For this review, take the finished solid that the model builds, in its own axes (mm). A direction names the side the tool comes from. Give positions to 0.01 mm unless a question says otherwise; leave off trailing zeros. Order: outer loops, then holes, each group sorted by start corner. A loop starts at its lowest first (then second) coordinate and runs counter-clockwise, first axis right, second up. Notation, with made-up numbers: M 55,-29.5 L 60,-29.5 A31 ccw 60,-3.5 Z; hole C -26,20.5 d2. An arc over 180 degrees is marked long. Use CSV: the item, a comma, the result in double quotes. Start each with the question number.
(1) Clearance check with flat-ended pins moving along their axes: P1, Ø4, axis at x = -5, z = 11, coming from the -Y side; P2, Ø6.5, axis at x = 15, z = -15, coming from the +Y side; P3, Ø2.5, axis at y = 3.5, z = -18, coming from the +X side. State where each tip first meets the part, or that it passes through.
(2) Draft analysis for pull direction Z (two halves, no side actions). For faces 4 (the face through (-23, 2, -25)), 5 (the face through (24.53, 2.54, 11.31)), 6 (the face through (-15.1, 2.5, -12.5)), 7 (the face through (-21, 2, 25)), state which applies: pulls with the +Z half, pulls with the -Z half, needs draft (parallel to the pull), parting line crosses it, or undercut.
(3) Tool access review of faces 1 (the face through (11.25, 2.535, -24.554)), 2 (the face through (18.69, 2.46, 24.53)), 3 (the face through (-25, 2, 2)): name each direction out of +Z, -Z, +X, -X, +Y, -Y from which nothing blocks a thin tool from reaching the whole face with its end or side.
(4) Consider section C-C (y = 3.65). Give the number of separate pieces and of enclosed holes in the cut face, and give its area (3 significant figures).
(5) Wall thickness on L1, parallel to X at y = 3.75, z = -15; L2, parallel to X at y = 1.4, z = 0; L3, parallel to Z at x = 0, y = 1.5: over which ranges is each line inside the solid? List them lowest first. Write a range as from..to.
(6) Consider section A-A (z = 16). Write out the cut boundary in (x, y).
(7) Consider section B-B (z = 3.5). Write out the cut boundary in (x, y).
```python
from build123d import *

# Parameters (mm, degrees)
SKETCH1_W           = 50
SKETCH1_H           = 50
SKETCH1_R           = 2.5
BOSS_EXTRUDE1_DEPTH = 5
SKETCH2_R           = 2.5
CUT_EXTRUDE1_DEPTH  = 5
CUT_EXTRUDE2_DEPTH  = 36.707142143
FILLET1_R           = 6


with BuildPart() as part:
    # Sketch1 → Boss-Extrude1 (new body)
    with BuildSketch(Plane(origin=(0, 0, 0), x_dir=(1, 0, 0), z_dir=(0, 1, 0))):
        Rectangle(SKETCH1_W, SKETCH1_H)
        with Locations(Location((15, 15, 0), (0, 0, 270))):
            Circle(SKETCH1_R, mode=Mode.SUBTRACT)
        with Locations(Location((15, -15, 0), (0, 0, 270))):
            Circle(SKETCH1_R, mode=Mode.SUBTRACT)
        with Locations(Location((-15, -15, 0), (0, 0, 90))):
            Circle(SKETCH1_R, mode=Mode.SUBTRACT)
        with Locations(Location((-15, 15, 0), (0, 0, 90))):
            Circle(SKETCH1_R, mode=Mode.SUBTRACT)
    extrude(amount=BOSS_EXTRUDE1_DEPTH)

    # Sketch2 → Cut-Extrude1 (cut)
    with BuildSketch(Plane(origin=(0, 5, 0), x_dir=(1, 0, 0), z_dir=(0, 1, 0))):
        with Locations((25, 15)):
            Circle(SKETCH2_R)
        with Locations((25, -15)):
            Circle(SKETCH2_R)
        with Locations((-25, 15)):
            Circle(SKETCH2_R)
        with Locations((-25, -15)):
            Circle(SKETCH2_R)
        with Locations((-15, 25)):
            Circle(SKETCH2_R)
        with Locations((15, 25)):
            Circle(SKETCH2_R)
        with Locations((15, -25)):
            Circle(SKETCH2_R)
        with Locations((-15, -25)):
            Circle(SKETCH2_R)
    extrude(amount=-CUT_EXTRUDE1_DEPTH, mode=Mode.SUBTRACT)

    # Sketch3 → Cut-Extrude2 (cut, through all)
    with BuildSketch(Plane(origin=(0, 5, 0), x_dir=(1, 0, 0), z_dir=(0, 1, 0))):
        with BuildLine():
            Line((-3, 19.696938457), (3, 19.696938457))
            Line((3, 19.696938457), (3, 14.696938457))
            ThreePointArc((3, 14.696938457), (0, -15), (-3, 14.696938457))
            Line((-3, 14.696938457), (-3, 19.696938457))
        make_face()
    extrude(amount=-CUT_EXTRUDE2_DEPTH, mode=Mode.SUBTRACT)

    # Fillet1
    fillet1_edges = [part.edges().sort_by_distance(p)[0] for p in [
        (-12.5, 2.5, 25),
        (17.5, 2.5, 25),
        (-25, 2.5, -12.5),
        (-25, 2.5, 17.5),
        (12.5, 2.5, -25),
        (-17.5, 2.5, -25),
        (25, 2.5, -17.5),
        (25, 2.5, 12.5),
    ]]
    fillet(fillet1_edges, radius=FILLET1_R)


solid = part.part
```
Check result:
1,P1,"passes through"
1,P2,"stops at y = 5"
1,P3,"stops at x = 24.73"
2,face 4,"pulls with the -Z half"
2,face 5,"undercut"
2,face 6,"undercut"
2,face 7,"pulls with the +Z half"
3,face 1,"-Z, +Y, -Y"
3,face 2,"+Z, +Y, -Y"
3,face 3,"+Z, -Z, -X, +Y, -Y"
4,separate pieces,"1"
4,enclosed holes,"5"
4,area,"1,600 mm^2"
5,L1,"x = -22.5..-17.5, -12.5..-3, 3..12.5, 17.5..22.5"
5,L2,"x = -25..-15, 15..25"
5,L3,"z = -25..-19.7, 15..25"
6,outline,"M -22.71,0 L -17.29,0 L -17.29,5 L -22.71,5 Z; M -12.71,0 L 12.71,0 L 12.71,5 L -12.71,5 Z; M 17.29,0 L 22.71,0 L 22.71,5 L 17.29,5 Z"
7,outline,"M -25,0 L -14.59,0 L -14.59,5 L -25,5 Z; M 14.59,0 L 25,0 L 25,5 L 14.59,5 Z"
